Could you check a few things on this model? Use its own coordinates, in mm. Face numbers are marked on the shaded views. A direction names the side the tool comes from. Coordinates: 2 decimals unless noted, no trailing zeros. Write each loop counter-clockwise with the first axis right and the second up, starting at its lowest first coordinate (ties: lowest second). Pieces come first, ordered by that corner, then holes.
```python
from build123d import *

# Parameters (mm, degrees)
EXTRUDE_1_DEPTH          = 4
SKETCH_2_R               = 10
CUT_EXTRUDE_1_DEPTH      = 2.5
EXTRUDE_4_DEPTH          = 2.5
CUT_EXTRUDE_2_DEPTH      = 127.614708745
CUT_EXTRUDE_2_DEPTH_BACK = 127.614708745
SKETCH_4_R               = 2.5
SKETCH_4_R_2             = 2.500304397
CHAMFER_1_SIZE           = 2.5
CHAMFER_2_SIZE           = 2.5
FILLET_1_R               = 10


with BuildPart() as part:
    # 草图1 → 凸台-拉伸1 (new, symmetric)
    with BuildSketch(Plane.XY):
        with BuildLine():
            Line((-2.397996919, 5.499964616), (-19.561052391, 8.526274367))
            Line((-19.561052391, 8.526274367), (-84.199167791, 0.661766964))
            Line((-84.199167791, 0.661766964), (-96.118365096, 5))
            Line((-96.118365096, 5), (-116.68337521, 5))
            ThreePointArc((-116.68337521, 5), (-126, 0), (-116.68337521, -5))
            Line((-116.68337521, -5), (-97.881634904, -5))
            Line((-97.881634904, -5), (-85.368824069, -9.554290691))
            Line((-85.368824069, -9.554290691), (-19.831257729, -1.58034726))
            Line((-19.831257729, -1.58034726), (-4.134478696, -4.348112914))
            ThreePointArc((-4.134478696, -4.348112914), (5.908846518, -1.041889066), (-2.397996919, 5.499964616))
        make_face()
    extrude(amount=EXTRUDE_1_DEPTH, both=True)

    # 草图2 → 切除-拉伸1 (cut)
    with BuildSketch(Plane(origin=(0, 0, -4), x_dir=(-1, 0, 0), z_dir=(0, 0, -1))):
        Circle(SKETCH_2_R)
    extrude(amount=-CUT_EXTRUDE_1_DEPTH, mode=Mode.SUBTRACT)

    # 草图3 → 凸台-拉伸4 (add)
    with BuildSketch(Plane.XY.offset(4)):
        with BuildLine():
            Line((-2.397996919, 5.499964616), (-7.660444431, 6.427876097))
            ThreePointArc((-7.660444431, 6.427876097), (-9.84807753, 1.736481777), (-9.396926208, -3.420201433))
            Line((-9.396926208, -3.420201433), (-4.134478696, -4.348112914))
            ThreePointArc((-4.134478696, -4.348112914), (5.908846518, -1.041889066), (-2.397996919, 5.499964616))
        make_face()
    extrude(amount=EXTRUDE_4_DEPTH)

    # 草图4 → 切除-拉伸2 (cut, two sides: drawn at the far end of the back side and taken through both)
    with BuildSketch(Plane(origin=(0, 0, -1.5), x_dir=(-1, 0, 0), z_dir=(0, 0, -1)).offset(-CUT_EXTRUDE_2_DEPTH_BACK)):
        Circle(SKETCH_4_R)
        with Locations((120, 0)):
            Circle(SKETCH_4_R_2)
    extrude(amount=CUT_EXTRUDE_2_DEPTH + CUT_EXTRUDE_2_DEPTH_BACK, mode=Mode.SUBTRACT)

    # 倒角1
    chamfer_1_edges = [part.edges().sort_by_distance(p)[0] for p in [
        (-9.84807753, 1.736481777, 4),
    ]]
    chamfer(chamfer_1_edges, length=CHAMFER_1_SIZE - 0.0001)  # a hair under: the kernel refuses the full size

    # 倒角2
    chamfer_2_edges = [part.edges().sort_by_distance(p)[0] for p in [
        (-9.84807753, 1.736481777, -1.5),
    ]]
    chamfer(chamfer_2_edges, length=CHAMFER_2_SIZE - 0.0001)  # a hair under: the kernel refuses the full size

    # 圆角1
    fillet_1_edges = [part.edges().sort_by_distance(p)[0] for p in [
        (-85.368824069, -9.554290691, 0),
        (-97.881634904, -5, 0),
        (-96.118365096, 5, 0),
        (-84.199167791, 0.661766964, 0),
    ]]
    fillet(fillet_1_edges, radius=FILLET_1_R)


solid = part.part
```
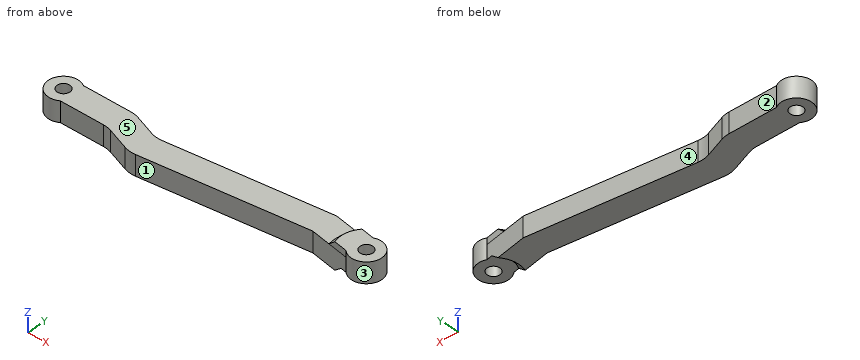
1. I want a section at D-D on x = -103. Please give me the cut outline in (y, z), plus the area to 3 significant figures.
Verdict:
outline: (-5, -4) - (5, -4) - (5, 4) - (-5, 4) - close
area: 80.0 mm2
2. I want a section at B-B on z = 1. Please give me the cut outline in (x, y), plus the area to 3 significant figures.
Verdict:
outline: (-116.68, -5) - (-99.64, -5) arc R10 cw to (-96.22, -5.6) - (-87.62, -8.74) arc R10 ccw to (-82.99, -9.27) - (-19.83, -1.58) - (-4.13, -4.35) arc R6 ccw (long way) to (-2.4, 5.5) - (-19.56, 8.53) - (-81.82, 0.95) arc R10 cw to (-86.45, 1.48) - (-94.46, 4.4) arc R10 ccw to (-97.88, 5) - (-116.68, 5) arc R6 ccw (long way) to start; hole circle Ø5 at (-120, 0); hole circle Ø5 at (0, 0)
area: 1,300 mm2
3. I want a section at A-A on x = 0. Please give me the cut outline in (y, z).
Verdict:
outline: (-6, -1.5) - (-2.5, -1.5) - (-2.5, 6.5) - (-6, 6.5) - close; (2.5, -1.5) - (6, -1.5) - (6, 6.5) - (2.5, 6.5) - close
4. Please list where these lines run through material, in increasing order: line 1 along X through (y, z) = (0, 3.5); line 2 along Y through (x, z) = (0, 2); line 3 along Z through (x, y) = (-39, 3).
Verdict:
line 1: x = -126 to -122.5, -117.5 to -2.5, 2.5 to 6
line 2: y = -6 to -2.5, 2.5 to 6
line 3: z = -4 to 4
5. If we mould it in two halves opening along X, with no side actions, what happens to the marked faces 4 and 5? For each: pulls with the +X half, pulls with the -X half, needs draft (parallel to the pull), parting line crosses it, or undercut.
Verdict:
face 4: undercut
face 5: needs draft
6. On a 3-axis mill with a long thin cutter (end or side, diameter ignored), from which of +Z, -Z, +X, -X, +Y, -Y can I reach the whole of each face in a straight line? I mean the marked faces 1, 2 and 3. Say none if no direction works.
Verdict:
face 1: +Z, -Z, -Y
face 2: +Z, -Z, +Y
face 3: +Z, -Z
7. I want a section at C-C on x = -120. Please give me the cut outline in (y, z).
Verdict:
outline: (-6, -4) - (-2.5, -4) - (-2.5, 4) - (-6, 4) - close; (2.5, -4) - (6, -4) - (6, 4) - (2.5, 4) - close
8. For pin 1 (5 mm diameter, centred on x = -25, z = -0.5, fed in from +Y); pin 2 (1 mm diameter, centred on y = 3.5, z = 2.5, fed in from -X); pin 3 (5 mm diameter, centred on y = 5.5, z = 0.5, fed in from +X); pin 4 (3 mm diameter, centred on x = 0, y = 0, fed in from -Z), each with a flat end and sliding along its axis, tell me the tip position at first contact or that it passes through.
Verdict:
pin 1: stops at y = 8.17
pin 2: stops at x = -125.2
pin 3: stops at x = 5.2
pin 4: passes through
